Verification items for the finished model (mm, model axes). Face numbers are marked on the shaded views. A direction names the side the tool comes from. Coordinates: 2 decimals unless noted, no trailing zeros. Write each loop counter-clockwise with the first axis right and the second up, starting at its lowest first coordinate (ties: lowest second). Pieces come first, ordered by that corner, then holes. Notation, with made-up numbers: M -19.75,11.5 L 24.25,11.5 A15 cw 24.25,34.5 Z; hole C 60,32.5 d8. An arc over 180 degrees is marked long. One line per item, written item: value.
```python
from build123d import *

# Parameters (mm, degrees)
SKETCH_1_W          = 44
SKETCH_1_H          = 25
EXTRUDE_1_DEPTH     = 2
SKETCH_2_W          = 2
SKETCH_2_H          = 25
EXTRUDE_2_DEPTH     = 56
FILLET_1_RADIUS     = 12.5
FILLET_1_LENGTH     = 2
CUT_EXTRUDE_2_REACH = 63.451
SKETCH_3_R          = 4.1
SKETCH_3_R_2        = 1.5
CUT_EXTRUDE_3_REACH = 74.307
SKETCH_4_R          = 4.1
SKETCH_4_R_2        = 1.5
FILLET_2_R          = 2


with BuildPart() as part:
    # 草图1 → 凸台-拉伸1 (new body)
    with BuildSketch(Plane(origin=(0, 0, 0), x_dir=(1, 0, 0), z_dir=(0, 1, 0))):
        Rectangle(SKETCH_1_W, SKETCH_1_H)
    extrude(amount=-EXTRUDE_1_DEPTH)

    # 草图2 → 凸台-拉伸2 (add)
    with BuildSketch(Plane(origin=(0, 0, 0), x_dir=(1, 0, 0), z_dir=(0, 1, 0))):
        with Locations((-21, 0)):
            Rectangle(SKETCH_2_W, SKETCH_2_H)
    extrude(amount=-EXTRUDE_2_DEPTH)

    # 圆角1: full round fillet: the end face becomes a half cylinder, R = half its width
    fillet_1_face = Plane((22, -1, 0), x_dir=(0, 1, 0), z_dir=(1, 0, 0))  # on the end face: x along it, z out of the body
    fillet_1_slab = fillet_1_face.offset(-FILLET_1_RADIUS / 2) * Box(FILLET_1_LENGTH, 2 * FILLET_1_RADIUS, FILLET_1_RADIUS, mode=Mode.PRIVATE)  # the body's end, R deep
    fillet_1_round = Plane((9.5, -1, 0), x_dir=(1, 0, 0), z_dir=(0, 1, 0)) * Cylinder(FILLET_1_RADIUS, FILLET_1_LENGTH, mode=Mode.PRIVATE)  # its axis R under the face
    add(fillet_1_slab - fillet_1_round, mode=Mode.SUBTRACT)

    # 草图3 → 切除-拉伸2 (cut, up to next)
    with BuildSketch(Plane(origin=(0, 0, 0), x_dir=(1, 0, 0), z_dir=(0, 1, 0)), mode=Mode.PRIVATE) as cut_extrude_2_sk1:
        with Locations(Location((9.5, 0, 0), (0, 0, 270))):
            Circle(SKETCH_3_R)
    cut_extrude_2_tool1 = extrude(cut_extrude_2_sk1.sketch, amount=-CUT_EXTRUDE_2_REACH, mode=Mode.PRIVATE) & part.part
    # 草图3 → 切除-拉伸2 (cut, up to next)
    with BuildSketch(Plane(origin=(0, 0, 0), x_dir=(1, 0, 0), z_dir=(0, 1, 0)), mode=Mode.PRIVATE) as cut_extrude_2_sk2:
        with Locations(Location((2.4, 0, 0), (0, 0, 270))):
            Circle(SKETCH_3_R_2)
    cut_extrude_2_tool2 = extrude(cut_extrude_2_sk2.sketch, amount=-CUT_EXTRUDE_2_REACH, mode=Mode.PRIVATE) & part.part
    # 草图3 → 切除-拉伸2 (cut, up to next)
    with BuildSketch(Plane(origin=(0, 0, 0), x_dir=(1, 0, 0), z_dir=(0, 1, 0)), mode=Mode.PRIVATE) as cut_extrude_2_sk3:
        with Locations(Location((9.5, 7.1, 0), (0, 0, 270))):
            Circle(SKETCH_3_R_2)
    cut_extrude_2_tool3 = extrude(cut_extrude_2_sk3.sketch, amount=-CUT_EXTRUDE_2_REACH, mode=Mode.PRIVATE) & part.part
    # 草图3 → 切除-拉伸2 (cut, up to next)
    with BuildSketch(Plane(origin=(0, 0, 0), x_dir=(1, 0, 0), z_dir=(0, 1, 0)), mode=Mode.PRIVATE) as cut_extrude_2_sk4:
        with Locations(Location((16.6, 0, 0), (0, 0, 270))):
            Circle(SKETCH_3_R_2)
    cut_extrude_2_tool4 = extrude(cut_extrude_2_sk4.sketch, amount=-CUT_EXTRUDE_2_REACH, mode=Mode.PRIVATE) & part.part
    # 草图3 → 切除-拉伸2 (cut, up to next)
    with BuildSketch(Plane(origin=(0, 0, 0), x_dir=(1, 0, 0), z_dir=(0, 1, 0)), mode=Mode.PRIVATE) as cut_extrude_2_sk5:
        with Locations(Location((9.5, -7.1, 0), (0, 0, 270))):
            Circle(SKETCH_3_R_2)
    cut_extrude_2_tool5 = extrude(cut_extrude_2_sk5.sketch, amount=-CUT_EXTRUDE_2_REACH, mode=Mode.PRIVATE) & part.part
    # 草图3 → 切除-拉伸2 (cut, up to next)
    with BuildSketch(Plane(origin=(0, 0, 0), x_dir=(1, 0, 0), z_dir=(0, 1, 0)), mode=Mode.PRIVATE) as cut_extrude_2_sk6:
        with Locations(Location((-9.2, 0, 0), (0, 0, 270))):
            Circle(SKETCH_3_R_2)
    cut_extrude_2_tool6 = extrude(cut_extrude_2_sk6.sketch, amount=-CUT_EXTRUDE_2_REACH, mode=Mode.PRIVATE) & part.part
    add(cut_extrude_2_tool1.solids().sort_by_distance((9.5, 0, 0))[0], mode=Mode.SUBTRACT)
    add(cut_extrude_2_tool2.solids().sort_by_distance((2.4, 0, 0))[0], mode=Mode.SUBTRACT)
    add(cut_extrude_2_tool3.solids().sort_by_distance((9.5, 0, -7.1))[0], mode=Mode.SUBTRACT)
    add(cut_extrude_2_tool4.solids().sort_by_distance((16.6, 0, 0))[0], mode=Mode.SUBTRACT)
    add(cut_extrude_2_tool5.solids().sort_by_distance((9.5, 0, 7.1))[0], mode=Mode.SUBTRACT)
    add(cut_extrude_2_tool6.solids().sort_by_distance((-9.2, 0, 0))[0], mode=Mode.SUBTRACT)

    # 镜向2: part across plane


with BuildPart() as part_1:
    add(part.part)
    add(part.part.mirror(Plane.ZX.offset(-28)))

    # 草图4 → 切除-拉伸3 (cut, up to next)
    with BuildSketch(Plane.ZY.offset(22), mode=Mode.PRIVATE) as cut_extrude_3_sk1:
        with Locations((0, -28)):
            Circle(SKETCH_4_R)
    cut_extrude_3_tool1 = extrude(cut_extrude_3_sk1.sketch, amount=-CUT_EXTRUDE_3_REACH, mode=Mode.PRIVATE) & part_1.part
    # 草图4 → 切除-拉伸3 (cut, up to next)
    with BuildSketch(Plane.ZY.offset(22), mode=Mode.PRIVATE) as cut_extrude_3_sk2:
        with Locations((0, -20.9)):
            Circle(SKETCH_4_R_2)
    cut_extrude_3_tool2 = extrude(cut_extrude_3_sk2.sketch, amount=-CUT_EXTRUDE_3_REACH, mode=Mode.PRIVATE) & part_1.part
    # 草图4 → 切除-拉伸3 (cut, up to next)
    with BuildSketch(Plane.ZY.offset(22), mode=Mode.PRIVATE) as cut_extrude_3_sk3:
        with Locations((7.1, -28)):
            Circle(SKETCH_4_R_2)
    cut_extrude_3_tool3 = extrude(cut_extrude_3_sk3.sketch, amount=-CUT_EXTRUDE_3_REACH, mode=Mode.PRIVATE) & part_1.part
    # 草图4 → 切除-拉伸3 (cut, up to next)
    with BuildSketch(Plane.ZY.offset(22), mode=Mode.PRIVATE) as cut_extrude_3_sk4:
        with Locations((0, -35.1)):
            Circle(SKETCH_4_R_2)
    cut_extrude_3_tool4 = extrude(cut_extrude_3_sk4.sketch, amount=-CUT_EXTRUDE_3_REACH, mode=Mode.PRIVATE) & part_1.part
    # 草图4 → 切除-拉伸3 (cut, up to next)
    with BuildSketch(Plane.ZY.offset(22), mode=Mode.PRIVATE) as cut_extrude_3_sk5:
        with Locations((-7.1, -28)):
            Circle(SKETCH_4_R_2)
    cut_extrude_3_tool5 = extrude(cut_extrude_3_sk5.sketch, amount=-CUT_EXTRUDE_3_REACH, mode=Mode.PRIVATE) & part_1.part
    # 草图4 → 切除-拉伸3 (cut, up to next)
    with BuildSketch(Plane.ZY.offset(22), mode=Mode.PRIVATE) as cut_extrude_3_sk6:
        with Locations((0, -6.9)):
            Circle(SKETCH_4_R_2)
    cut_extrude_3_tool6 = extrude(cut_extrude_3_sk6.sketch, amount=-CUT_EXTRUDE_3_REACH, mode=Mode.PRIVATE) & part_1.part
    # 草图4 → 切除-拉伸3 (cut, up to next)
    with BuildSketch(Plane.ZY.offset(22), mode=Mode.PRIVATE) as cut_extrude_3_sk7:
        with Locations(Location((0, -49.1, 0), (0, 0, 180))):
            Circle(SKETCH_4_R_2)
    cut_extrude_3_tool7 = extrude(cut_extrude_3_sk7.sketch, amount=-CUT_EXTRUDE_3_REACH, mode=Mode.PRIVATE) & part_1.part
    add(cut_extrude_3_tool1.solids().sort_by_distance((-22, -28, 0))[0], mode=Mode.SUBTRACT)
    add(cut_extrude_3_tool2.solids().sort_by_distance((-22, -20.9, 0))[0], mode=Mode.SUBTRACT)
    add(cut_extrude_3_tool3.solids().sort_by_distance((-22, -28, 7.1))[0], mode=Mode.SUBTRACT)
    add(cut_extrude_3_tool4.solids().sort_by_distance((-22, -35.1, 0))[0], mode=Mode.SUBTRACT)
    add(cut_extrude_3_tool5.solids().sort_by_distance((-22, -28, -7.1))[0], mode=Mode.SUBTRACT)
    add(cut_extrude_3_tool6.solids().sort_by_distance((-22, -6.9, 0))[0], mode=Mode.SUBTRACT)
    add(cut_extrude_3_tool7.solids().sort_by_distance((-22, -49.1, 0))[0], mode=Mode.SUBTRACT)

    # 圆角2
    fillet_2_edges = [part_1.edges().sort_by_distance(p)[0] for p in [
        (-22, -56, 0),
        (-22, 0, 0),
    ]]
    fillet(fillet_2_edges, radius=FILLET_2_R)


solid = part_1.part
```
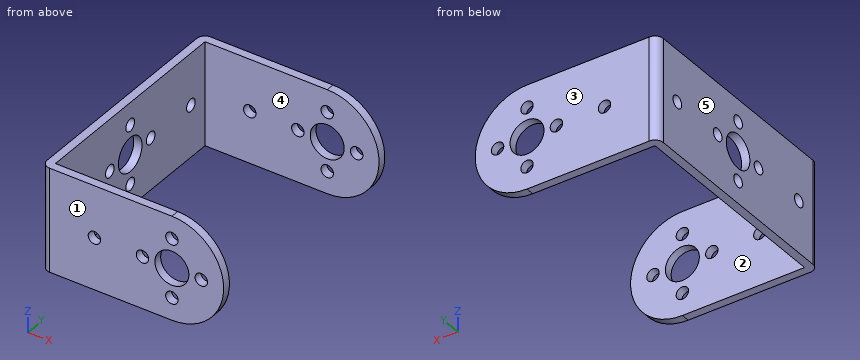
Item 1: Cross-section at B-B, the plane x = -13. Enter the section's corners in (y, z), and give its area (3 significant figures).
The answers:
outline: M -56,-12.5 L -54,-12.5 L -54,12.5 L -56,12.5 Z; M -2,-12.5 L 0,-12.5 L 0,12.5 L -2,12.5 Z
area: 100 mm²
Item 2: Cross-section at A-A, the plane y = -28. Enter the section's corners in (x, z).
The answers:
outline: M -22,-12.5 L -20,-12.5 L -20,-8.6 L -22,-8.6 Z; M -22,-5.6 L -20,-5.6 L -20,-4.1 L -22,-4.1 Z; M -22,4.1 L -20,4.1 L -20,5.6 L -22,5.6 Z; M -22,8.6 L -20,8.6 L -20,12.5 L -22,12.5 Z
Item 3: Cross-section at C-C, the plane z = -6.25. Enter the section's corners in (x, y).
The answers:
outline: M -22,-54 A2 ccw -20,-56 L 8.26,-56 L 8.26,-54 L -20,-54 L -20,-29.24 L -22,-29.24 Z; M -22,-26.76 L -20,-26.76 L -20,-2 L 8.26,-2 L 8.26,0 L -20,0 A2 ccw -22,-2 Z; M 10.74,-56 L 20.33,-56 L 20.33,-54 L 10.74,-54 Z; M 10.74,-2 L 20.33,-2 L 20.33,0 L 10.74,0 Z
Item 4: Go/stop test with a flat-tipped pin: P1, Ø5, axis at y = -44, z = 2, coming from the +X side. Record where the tip stops, or that it passes through.
The answers:
P1: stops at x = -20
Item 5: Scan lines: line 1 (Z direction, x = -20.55, y = -49.1); line 2 (Y direction, x = 17, z = -5); line 3 (X direction, y = -54.8, z = 0). Record each from-to range of solid material in increasing order.
The answers:
line 1: z = -12.5 to -1.5, 1.5 to 12.5
line 2: y = -56 to -54, -2 to 0
line 3: x = -21.83 to -10.7, -7.7 to 0.9, 3.9 to 5.4, 13.6 to 15.1, 18.1 to 22
Item 6: Cross-section at D-D, the plane y = -49.1. Enter the section's corners in (x, z).
The answers:
outline: M -22,-12.5 L -20,-12.5 L -20,-1.5 L -22,-1.5 Z; M -22,1.5 L -20,1.5 L -20,12.5 L -22,12.5 Z
Item 7: Draft check along Y on the marked faces 1, 2 and 3. Enter one of: released by +Y, released by -Y, zero draft, split by the parting line, or undercut.
The answers:
face 1: released by -Y
face 2: undercut
face 3: released by +Y
Item 8: Access from +Z, -Z, +X, -X, +Y, -Y to the whole of each face (thin tool, end or side, straight path). Record for the marked faces 4 and 5.
The answers:
face 4: +Z, -Z, +X
face 5: +Z, -Z, -X, +Y, -Y
